```python
from build123d import *

# Parameters (mm, degrees)
SKETCH1_R           = 14
BOSS_EXTRUDE1_DEPTH = 100
SKETCH2_R           = 18
BOSS_EXTRUDE2_DEPTH = 5
SKETCH3_R           = 3
BOSS_EXTRUDE3_DEPTH = 20


with BuildPart() as part:
    # Sketch1 → Boss-Extrude1 (new body)
    with BuildSketch(Plane(origin=(0, 0, 0), x_dir=(1, 0, 0), z_dir=(0, 1, 0))):
        Circle(SKETCH1_R)
    extrude(amount=BOSS_EXTRUDE1_DEPTH)

    # Sketch2 → Boss-Extrude2 (add)
    with BuildSketch(Plane(origin=(0, 100, 0), x_dir=(1, 0, 0), z_dir=(0, 1, 0))):
        Circle(SKETCH2_R)
    extrude(amount=BOSS_EXTRUDE2_DEPTH)

    # Sketch3 → Boss-Extrude3 (add)
    with BuildSketch(Plane(origin=(0, 105, 0), x_dir=(1, 0, 0), z_dir=(0, 1, 0))):
        Circle(SKETCH3_R)
    extrude(amount=BOSS_EXTRUDE3_DEPTH)


solid = part.part
```
Geometry: final body of the model. Coordinates: model frame, mm. A direction names the side the tool comes from. Round coordinates to 2 decimals unless told otherwise and drop trailing zeros. Order: outer loops, then holes, each group sorted by start corner. A loop starts at its lowest first (then second) coordinate and runs counter-clockwise, first axis right, second up. Notation, with made-up numbers: (-20, 23) - (1, 23) arc R29 ccw to (1, 52) - close; hole circle Ø3 at (-29, 36). An arc over 180 degrees is marked (long way). Write item = value, one per line. Start each with the question number.
Q1. Cut plane B-B on z = 0. Return the cut outline in (x, y).
Q2. Cut plane A-A on x = -9. Return the cut outline in (y, z), and give its area (3 significant figures).
Q3. Access query for faces 1 (the flat face through (9, 100, 11)), 2 (the cylindrical face through (-3, 115, 0)), 3 (the flat face through (0, 125, 0)). Directions: +Z, -Z, +X, -X, +Y, -Y. A direction counts if a zero-diameter tool reaches every point of the face in a straight line with its end or side. Return the directions, or none.
Q4. Ray query, line 1 (Y direction, x = -14, z = 2.5); line 2 (Y direction, x = -7, z = -6); line 3 (X direction, y = 102, z = -0.5). Return the intervals inside material, ascending. Write a range as from..to.
Q5. Cut plane D-D on x = 0. Return the cut outline in (y, z), and give its area (3 significant figures).
Q6. Pin query (flat end, axial travel): pin 1 (8 mm diameter, centred on y = 30.5, z = -11, fed in from -X); pin 2 (4 mm diameter, centred on y = 59, z = -3, fed in from +X); pin 3 (2 mm diameter, centred on y = 71, z = -1, fed in from -X). Return the tip coordinate at first contact, or that it passes through.
Q7. Cut plane C-C on y = 20.5. Return the cut outline in (x, z), and give its area (3 significant figures).
Outcome:
q1.outline = (-18, 100) - (-14, 100) - (-14, 0) - (14, 0) - (14, 100) - (18, 100) - (18, 105) - (3, 105) - (3, 125) - (-3, 125) - (-3, 105) - (-18, 105) - close
q2.outline = (0, -10.72) - (100, -10.72) - (100, -15.59) - (105, -15.59) - (105, 15.59) - (100, 15.59) - (100, 10.72) - (0, 10.72) - close
q2.area = 2,300 mm^2
q3.face_1 = -Y
q3.face_2 = +Y
q3.face_3 = +Z, -Z, +X, -X, +Y
q4.line_1 = 100..105
q4.line_2 = 0..105
q4.line_3 = -17.99..17.99
q5.outline = (0, -14) - (100, -14) - (100, -18) - (105, -18) - (105, -3) - (125, -3) - (125, 3) - (105, 3) - (105, 18) - (100, 18) - (100, 14) - (0, 14) - close
q5.area = 3,100 mm^2
q6.pin_1 = -12.12
q6.pin_2 = 13.96
q6.pin_3 = -14
q7.outline = circle Ø28 at (0, 0)
q7.area = 616 mm^2
